CAD build for the part. Positions are in the model's coordinates, mm. Give positions to 0.01 mm unless a question says otherwise; leave off trailing zeros. Write each loop counter-clockwise with the first axis right and the second up, starting at its lowest first coordinate (ties: lowest second). Pieces come first, ordered by that corner, then holes. Notation, with made-up numbers: (48.5, 20.5) -> (77.5, 20.5) arc R29 cw to (77.5, 48.5) -> close; hole circle Ø3 at (-21, -22.5). An arc over 180 degrees is marked (long way). Answer in a Markdown table with one row per item. Add a question column.
```python
from build123d import *

# Parameters (mm, degrees)
CSK_FOR_M4_HEX_SOCKET_COUNTERSUNK_HE_2_COUNT = 2
CSK_FOR_M4_HEX_SOCKET_COUNTERSUNK_HE_2_PITCH = 46
FILLET1_R                                    = 1
CHAMFER1_SIZE                                = 0.5
SKETCH6_R                                    = 20.074468172
CUT_EXTRUDE2_DEPTH                           = 10


with BuildPart() as part:
    # Sketch1 → Revolve1 (revolve)
    with BuildSketch(Plane.XY, mode=Mode.PRIVATE) as revolve1_sk:
        Polygon((-30, -2), (-30, 2), (-16, 2), (-16, 4), (-13, 4), (-13, -2), align=None)
    revolve(revolve1_sk.sketch.rotate(Axis((0, 55, 0), (0, -1, 0)), 270), axis=Axis((0, 55, 0), (0, -1, 0)))

    # Sketch3 → CSK for M4 Hex Socket Countersunk Head Screw2 (revolve, cut)
    with BuildSketch(Plane(origin=(0, -2, 23), x_dir=(0, 0, -1), z_dir=(1, 0, 0))):
        Polygon((0, 0), (0, 4), (2.25, 4), (2.25, 2.34), (4.59, 0), align=None)
    csk_for_m4_hex_socket_countersunk_head_s = revolve(axis=Axis((0, -8.35, 23), (0, 1, 0)), mode=Mode.SUBTRACT)

    # CSK for M4 Hex Socket Countersunk He 2: CSK for M4 Hex Socket Countersunk Head Screw2 ×2
    with Locations(*[(0, 0, -i * CSK_FOR_M4_HEX_SOCKET_COUNTERSUNK_HE_2_PITCH) for i in range(1, CSK_FOR_M4_HEX_SOCKET_COUNTERSUNK_HE_2_COUNT)]):
        add(csk_for_m4_hex_socket_countersunk_head_s, mode=Mode.SUBTRACT)

    # Fillet1
    fillet1_edges = [part.edges().sort_by_distance(p)[0] for p in [
        (0, -2, -13),
    ]]
    fillet(fillet1_edges, radius=FILLET1_R)

    # Chamfer1
    chamfer1_edges = [part.edges().sort_by_distance(p)[0] for p in [
        (0, 4, -16),
    ]]
    chamfer(chamfer1_edges, length=CHAMFER1_SIZE)

    # Sketch6 → Cut-Extrude2 (cut)
    with BuildSketch(Plane(origin=(0, 2, 0), x_dir=(1, 0, 0), z_dir=(0, 1, 0))):
        Circle(SKETCH6_R)
    extrude(amount=CUT_EXTRUDE2_DEPTH, mode=Mode.SUBTRACT)


solid = part.part
```
Item 1: Slice it at B-B, the plane x = 0. List the corners of the cut face in (y, z), then the cut area to 3 significant figures.
Item 2: Slice it at A-A, the plane z = 0. List the corners of the cut face in (x, y), then the cut area to 3 significant figures.
Item 3: Mould opens along X. For faces 1 (the face through (2.339, 0.194, 23.519)), 2 (the face through (6, 2, 13)), 3 (the face through (-1.32, 0.03, -29.97)) say: released by +X, released by -X, zero draft, split by the parting line, or undercut.
Item 4: Probe L1, parallel to X at y = 0.9, z = 0; L2, parallel to X at y = 1.45, z = 23; L3, parallel to Z at x = 6.5, y = 1.45. List the from-to ranges inside material, lowest first. Write a range as from..to.
Item 5: Drop flat-ended pins along their axis: pin 1 Ø2 at (x, y) = (8, -0.5) entering from +Z; pin 2 Ø3.5 at (x, z) = (0, 23) entering from -Y; pin 3 Ø1 at (y, z) = (1, -4.5) entering from -X; pin 4 Ø1.5 at (y, z) = (0, 1) entering from -X. Give the stop position or say it passes through.
Item 6: Slice it at D-D, the plane x = 26. List the corners of the cut face in (y, z), then the cut area to 3 significant figures.
Item 7: Slice it at C-C, the plane z = -23. List the corners of the cut face in (x, y).
Answer key:
| question | item | result |
|---|---|---|
| 1 | outline | (-2, -30) -> (2, -30) -> (2, -25.25) -> (0.34, -25.25) -> (-2, -27.59) -> close; (-2, -18.41) -> (0.34, -20.75) -> (2, -20.75) -> (2, -13) -> (-1, -13) arc R1 ccw to (-2, -14) -> close; (-2, 14) arc R1 ccw to (-1, 13) -> (2, 13) -> (2, 20.75) -> (0.34, 20.75) -> (-2, 18.41) -> close; (-2, 27.59) -> (0.34, 25.25) -> (2, 25.25) -> (2, 30) -> (-2, 30) -> close |
| 1 | area | 88.6 mm² |
| 2 | outline | (-30, -2) -> (-14, -2) arc R1 ccw to (-13, -1) -> (-13, 2) -> (-30, 2) -> close; (13, -1) arc R1 ccw to (14, -2) -> (30, -2) -> (30, 2) -> (13, 2) -> close |
| 2 | area | 136 mm² |
| 3 | face 1 | undercut |
| 3 | face 2 | zero draft |
| 3 | face 3 | split by the parting line |
| 4 | L1 | x = -30..-13, 13..30 |
| 4 | L2 | x = -19.26..-2.25, 2.25..19.26 |
| 4 | L3 | z = -29.29..-11.26, 11.26..29.29 |
| 5 | pin 1 | stops at z = 29.17 |
| 5 | pin 2 | passes through |
| 5 | pin 3 | stops at x = -29.73 |
| 5 | pin 4 | stops at x = -30 |
| 6 | outline | (-2, -14.97) -> (2, -14.97) -> (2, 14.97) -> (-2, 14.97) -> close |
| 6 | area | 120 mm² |
| 7 | outline | (-19.26, -2) -> (-4.59, -2) -> (-2.25, 0.34) -> (-2.25, 2) -> (-19.26, 2) -> close; (2.25, 0.34) -> (4.59, -2) -> (19.26, -2) -> (19.26, 2) -> (2.25, 2) -> close |
